Autodesk Inventor part; units mm, degrees
ref_plane "YZ Plane" through (0, 0, 0) normal (1, 0, 0) x (0, 1, 0)
ref_plane "XZ Plane" through (0, 0, 0) normal (0, 1, 0) x (-1, 0, 0)
ref_plane "XY Plane" through (0, 0, 0) normal (0, 0, 1) x (1, 0, 0)
sketch "Эскиз1" plane through (0, 0, 0) normal (0, 0, 1) x (1, 0, 0)
  line L0 (7, -2) -> (-7, -2)
  line L1 (-7, -2) -> (-7, 2)
  line L2 (-7, 2) -> (7, 2)
  line L3 (7, 2) -> (7, -2)
  line L4 (7, -2) -> (-7, 2) construction
  line L5 (-7, -2) -> (7, 2) construction
  line L6 (4, -2) -> (-4, -2)
  line L7 (-4, -2) -> (-4, 2)
  line L8 (-4, 2) -> (4, 2)
  line L9 (4, 2) -> (4, -2)
  line L10 (4, -2) -> (-4, 2) construction
  line L11 (-4, -2) -> (4, 2) construction
  line L12 (6.5, -1.5) -> (4.5, -1.5)
  line L13 (4.5, -2) -> (4.5, 2)
  line L14 (4.5, 1.5) -> (6.5, 1.5)
  line L15 (6.5, 2) -> (6.5, -2)
  line L16 (6.5, -1.5) -> (4.5, 1.5) construction
  line L17 (4.5, -1.5) -> (6.5, 1.5) construction
  line L18 (0, -2) -> (0, 2) construction
  point P0 (0, 0)
  point P1 (5.5, 0)
  dimension "d1" = 14
  dimension "d2" = 8
  dimension "d3" = 4
  dimension "d4" = 0.5
  dimension "d5" = 0.5
  dimension "d6" = 0.5
  dimension "d7" = 0.5
revolve "Вращение1" add sketch "Эскиз1" angle 360 about axis through (0, -2, 0) along (0, 1, 0) contours L0 L15 L2 L3 | L0 L9 L2 L13 | L12 L13 L14 L15
equation "\"d4\" = d6"
equation "\"d6\" = d7"
equation "\"d7\" = d5"
properties part number "Подшипник 8х14х4"
Could you check a few things on this model? Use its own coordinates, in mm. A direction names the side the tool comes from. Coordinates: 2 decimals unless noted, no trailing zeros. Order: outer loops, then holes, each group sorted by start corner. A loop starts at its lowest first (then second) coordinate and runs counter-clockwise, first axis right, second up. Notation, with made-up numbers: (58, 51.5) -> (63, 51.5) arc R25 ccw to (63, 81.5) -> close; hole circle Ø8 at (39, -8.5). An arc over 180 degrees is marked (long way). One line per item, written item: value. Start each with the question number.
1) I'm going to push flat-ended pins straight in: pin 1 (1 mm diameter, centred on x = -1.5, y = -1, fed in from -Z); pin 2 (1.5 mm diameter, centred on x = -4.5, y = 1.5, fed in from +Z); pin 3 (1 mm diameter, centred on x = -5.5, y = -0.5, fed in from -Z). Where does each tip first touch, or does it pass through?
2) Imagine slicing it at B-B on x = 0. List the corners of the cut face in (y, z) for me.
3) Imagine slicing it at D-D on z = 4.25. List the corners of the cut face in (x, y) for me.
4) Imagine slicing it at A-A on z = 0. List the corners of the cut face in (x, y) for me.
5) Which directions (+Z, -Z, +X, -X, +Y, -Y) give clear straight access to the entire face, cutting with the end or side of a thin tool? Please do faces 4 (the cylindrical face through (-5.158, 1.746, -3.955)), 5 (the flat face through (-1.54, -1.5, -4.42)), 6 (the flat face through (-3, 2, 3)).
6) Imagine slicing it at C-C on y = -0.9. List the corners of the cut face in (x, z) for me, plus the area to 3 significant figures.
7) We'd pull the mould along Z, two halves only. Please class faces 1 (the flat face through (-3, -2, 3)), 2 (the cylindrical face through (-0.867, -0.028, -3.905)), 3 (the cylindrical face through (6.466, -0.028, -2.681)): +Z half, -Z half, draft (parallel to the pull), parting line (faces both ways), or undercut.
8) If I drill on L1, parallel to X at y = -1.8, z = 0; L2, parallel to X at y = 0.2, z = 0, over which ranges is the centre line in solid material (lowest first)? Write a range as [from, to].
Answer list:
1. pin 1: stops at z = -6.93
1. pin 2: stops at z = 5.91
1. pin 3: stops at z = -4.9
2. outline: (-2, -7) -> (2, -7) -> (2, -6.5) -> (1.5, -6.5) -> (1.5, -4.5) -> (2, -4.5) -> (2, -4) -> (-2, -4) -> (-2, -4.5) -> (-1.5, -4.5) -> (-1.5, -6.5) -> (-2, -6.5) -> close; (-2, 4) -> (2, 4) -> (2, 4.5) -> (1.5, 4.5) -> (1.5, 6.5) -> (2, 6.5) -> (2, 7) -> (-2, 7) -> (-2, 6.5) -> (-1.5, 6.5) -> (-1.5, 4.5) -> (-2, 4.5) -> close
3. outline: (-5.56, -2) -> (-4.92, -2) -> (-4.92, -1.5) -> (-1.48, -1.5) -> (-1.48, -2) -> (1.48, -2) -> (1.48, -1.5) -> (4.92, -1.5) -> (4.92, -2) -> (5.56, -2) -> (5.56, 2) -> (4.92, 2) -> (4.92, 1.5) -> (1.48, 1.5) -> (1.48, 2) -> (-1.48, 2) -> (-1.48, 1.5) -> (-4.92, 1.5) -> (-4.92, 2) -> (-5.56, 2) -> close
4. outline: (-7, -2) -> (-6.5, -2) -> (-6.5, -1.5) -> (-4.5, -1.5) -> (-4.5, -2) -> (-4, -2) -> (-4, 2) -> (-4.5, 2) -> (-4.5, 1.5) -> (-6.5, 1.5) -> (-6.5, 2) -> (-7, 2) -> close; (4, -2) -> (4.5, -2) -> (4.5, -1.5) -> (6.5, -1.5) -> (6.5, -2) -> (7, -2) -> (7, 2) -> (6.5, 2) -> (6.5, 1.5) -> (4.5, 1.5) -> (4.5, 2) -> (4, 2) -> close
5. face 4: +Y
5. face 5: -Y
5. face 6: +Z, -Z, +X, -X, +Y
6. outline: circle Ø14 at (0, 0); hole circle Ø8 at (0, 0)
6. area: 104 mm2
7. face 1: draft
7. face 2: undercut
7. face 3: parting line
8. L1: x = [-7, -6.5], [-4.5, -4], [4, 4.5], [6.5, 7]
8. L2: x = [-7, -4], [4, 7]
